Work out the finished part from the listing and answer in its coordinate system (mm). Give positions to 0.01 mm unless a question says otherwise; leave off trailing zeros. Write each loop counter-clockwise with the first axis right and the second up, starting at its lowest first coordinate (ties: lowest second). Pieces come first, ordered by that corner, then holes.
1) Given pin 1 Ø3 at (y, z) = (18.29, 50.84) entering from -X, flat-ended and moving along its own axis, determine where the tip first touches the part or whether it passes through.
2) Straight lines are drawn through the part: probe 1 along Z at (x, y) = (-0.5, 3.5); probe 2 along Y at (x, z) = (-0.85, 46); probe 3 along Z at (x, y) = (-0.2, 2.5). For each, find the intervals that lie inside material, in ascending order.
3) Find section C-C (x = -1.75). Determine the outline of the cut face in (y, z), plus the area to 3 significant figures.
4) Find section D-D (y = -6). Determine the outline of the cut face in (x, z) (3 decimals).
5) Find section A-A (y = 8.89). Determine the outline of the cut face in (x, z) (3 decimals), plus the area to 3 significant figures.
6) Find section B-B (y = 13). Determine the outline of the cut face in (x, z) (3 decimals), plus the area to 3 significant figures.
```python
from build123d import *

# Parameters (mm, degrees)
BOSS_EXTRUDE1_DEPTH              = 3.175
F_10_0_1935_DIAMETER_HOLE1_D     = 4.9149
F_10_0_1935_DIAMETER_HOLE1_DEPTH = 11.176
F_10_0_1935_DIAMETER_HOLE1_TIP   = 1.476584928
SKETCH6_W                        = 3.175
SKETCH6_H                        = 19.05
SKETCH6_H_2                      = 12.7
CUT_EXTRUDE1_DEPTH               = 63.157515949
FILLET1_R                        = 3.81


with BuildPart() as part:
    # Sketch1 → Boss-Extrude1 (new body)
    with BuildSketch(Plane(origin=(0, 0, 0), x_dir=(0, 0, -1), z_dir=(1, 0, 0))):
        with BuildLine():
            Line((-11.43, 25.4), (-56.642, 25.4))
            Line((-56.642, 25.4), (-56.642, -12.13104))
            Line((-56.642, -12.13104), (-39.203469383, -12.13104))
            Line((-39.203469383, -12.13104), (-38.998073701, -12.13104))
            ThreePointArc((-38.998073701, -12.13104), (-37.012948259, -11.974934012), (-35.076624386, -11.510453697))
            Line((-35.076624386, -11.510453697), (-11.43, -3.833836163))
            Line((-11.43, -3.833836163), (-11.43, 25.4))
        make_face()
    extrude(amount=-BOSS_EXTRUDE1_DEPTH)

    # #10 (0.1935) Diameter Hole1
    with Locations(Plane(origin=(0, 0, 0), x_dir=(0, 0, -1), z_dir=(1, 0, 0))):
        with Locations((-50.8381, -5.08), (-50.8381, 18.288), (-32.512, 8.89)):
            Hole(F_10_0_1935_DIAMETER_HOLE1_D / 2, depth=F_10_0_1935_DIAMETER_HOLE1_DEPTH)
            with Locations((0, 0, -(F_10_0_1935_DIAMETER_HOLE1_DEPTH + F_10_0_1935_DIAMETER_HOLE1_TIP / 2))):  # 118° drill point
                Cone(0, F_10_0_1935_DIAMETER_HOLE1_D / 2, F_10_0_1935_DIAMETER_HOLE1_TIP, mode=Mode.SUBTRACT)

    # Sketch6 → Cut-Extrude1 (cut, through all)
    with BuildSketch(Plane.ZY.offset(3.175)):
        with Locations((44.6786, 6.223)):
            Rectangle(SKETCH6_W, SKETCH6_H)
        with Locations((20.364644497, 9.020993871)):
            Rectangle(SKETCH6_W, SKETCH6_H_2)
    extrude(amount=-CUT_EXTRUDE1_DEPTH, mode=Mode.SUBTRACT)

    # Fillet1
    fillet1_edges = [part.edges().sort_by_distance(p)[0] for p in [
        (-1.5875, -12.13104, 56.642),
        (-1.5875, 25.4, 56.642),
        (-1.5875, 25.4, 11.43),
        (-1.5875, -3.833836163, 11.43),
    ]]
    fillet(fillet1_edges, radius=FILLET1_R)


solid = part.part
```
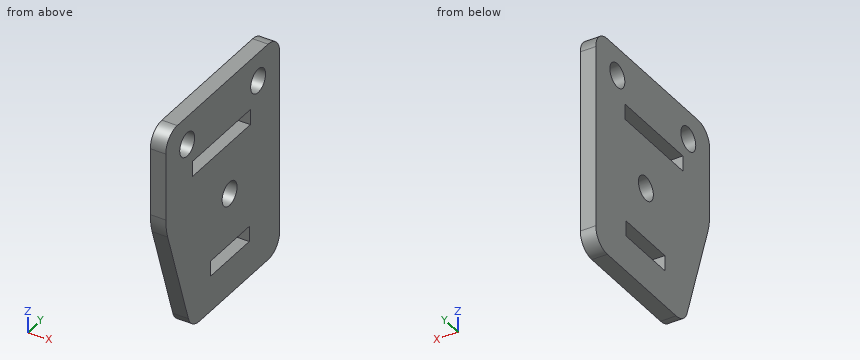
Results:
1. pin 1: passes through
2. probe 1: z = 11.43 to 18.78, 21.95 to 43.09, 46.27 to 56.64
2. probe 2: y = -12.13 to -3.3, 15.75 to 25.4
2. probe 3: z = 11.43 to 43.09, 46.27 to 56.64
3. outline: (-12.13, 39) arc R12.7 ccw to (-11.51, 35.08) - (-4.69, 14.06) arc R3.81 ccw to (-1.06, 11.43) - (21.59, 11.43) arc R3.81 ccw to (25.4, 15.24) - (25.4, 52.83) arc R3.81 ccw to (21.59, 56.64) - (-8.32, 56.64) arc R3.81 ccw to (-12.13, 52.83) - close; hole circle Ø4.91 at (-5.08, 50.84); hole (-3.3, 43.09) - (15.75, 43.09) - (15.75, 46.27) - (-3.3, 46.27) - close; hole (2.67, 18.78) - (15.37, 18.78) - (15.37, 21.95) - (2.67, 21.95) - close; hole circle Ø4.91 at (8.89, 32.51); hole circle Ø4.91 at (18.29, 50.84)
3. area: 1,420 mm2
4. outline: (-3.175, 18.103) - (0, 18.103) - (0, 48.559) - (-3.175, 48.559) - close; (-3.175, 53.117) - (0, 53.117) - (0, 56.642) - (-3.175, 56.642) - close
5. outline: (-3.175, 11.43) - (0, 11.43) - (0, 18.777) - (-3.175, 18.777) - close; (-3.175, 21.952) - (0, 21.952) - (0, 30.055) - (-3.175, 30.055) - close; (-3.175, 34.969) - (0, 34.969) - (0, 43.091) - (-3.175, 43.091) - close; (-3.175, 46.266) - (0, 46.266) - (0, 56.642) - (-3.175, 56.642) - close
5. area: 108 mm2
6. outline: (-3.175, 11.43) - (0, 11.43) - (0, 18.777) - (-3.175, 18.777) - close; (-3.175, 21.952) - (0, 21.952) - (0, 43.091) - (-3.175, 43.091) - close; (-3.175, 46.266) - (0, 46.266) - (0, 56.642) - (-3.175, 56.642) - close
6. area: 123 mm2
